```python
from build123d import *

# Parameters (mm, degrees)
SKETCH_1_R                       = 1.85
SKETCH_1_R_2                     = 32.5
SM_BASE_FLANGE_1_DEPTH           = 3
SM_EDGE_FLANGE_1_STRIP_W         = 13.4732
SM_EDGE_FLANGE_1_STRIP_H         = 3
SM_EDGE_FLANGE_1_STRIP_CUT_DEPTH = 100
SM_EDGE_FLANGE_1_DEPTH           = 100
SKETCH_9_R                       = 2.1
CUT_EXTRUDE_1_DEPTH              = 10
FILLET_1_R                       = 5
SKETCH_10_R                      = 2.1
CUT_EXTRUDE_2_DEPTH              = 10


# Sheet-metal steps are written as plain solids
with BuildPart() as part:
    # Sketch 1 → 基体-法兰1 (new body)
    with BuildSketch(Plane(origin=(0, 0, 0), x_dir=(0, 0, -1), z_dir=(1, 0, 0))):
        with BuildLine():
            Line((-50, 0), (-50, -55.5))
            Line((-50, -55.5), (50, -55.5))
            Line((50, -55.5), (50, 0))
            ThreePointArc((50, 0), (0, 50), (-50, 0))
        make_face()
        with Locations((0, 42.5)):
            Circle(SKETCH_1_R, mode=Mode.SUBTRACT)
        with Locations((30.0520382, 30.0520382)):
            Circle(SKETCH_1_R, mode=Mode.SUBTRACT)
        with Locations((42.5, 0)):
            Circle(SKETCH_1_R, mode=Mode.SUBTRACT)
        with Locations((30.0520382, -30.0520382)):
            Circle(SKETCH_1_R, mode=Mode.SUBTRACT)
        with Locations((0, -42.5)):
            Circle(SKETCH_1_R, mode=Mode.SUBTRACT)
        with Locations((-30.0520382, -30.0520382)):
            Circle(SKETCH_1_R, mode=Mode.SUBTRACT)
        with Locations((-42.5, 0)):
            Circle(SKETCH_1_R, mode=Mode.SUBTRACT)
        with Locations((-30.0520382, 30.0520382)):
            Circle(SKETCH_1_R, mode=Mode.SUBTRACT)
        Circle(SKETCH_1_R_2, mode=Mode.SUBTRACT)
    extrude(amount=-SM_BASE_FLANGE_1_DEPTH)

    # 边线-法兰1 strip (across the edge) → 边线-法兰1 strip cut (cut)
    with BuildSketch(Plane(origin=(-3, -55.5, -50), x_dir=(0, 1, 0), z_dir=(0, 0, 1))):
        with Locations((-3, -1.5)):
            Rectangle(SM_EDGE_FLANGE_1_STRIP_W, SM_EDGE_FLANGE_1_STRIP_H)
    extrude(amount=SM_EDGE_FLANGE_1_STRIP_CUT_DEPTH, mode=Mode.SUBTRACT)

    # 边线-法兰1 section (across the edge) → 边线-法兰1 (add)
    with BuildSketch(Plane(origin=(-3, -55.5, -50), x_dir=(0, 1, 0), z_dir=(0, 0, 1))):
        with BuildLine():
            Line((0, 0.7366), (0, 50))
            Line((0, 50), (3, 50))
            Line((3, 50), (3, 0.7366))
            ThreePointArc((3, 0.7366), (3.215745145, 0.215745145), (3.7366, 0))
            Line((3.7366, 0), (3.7366, -3))
            ThreePointArc((3.7366, -3), (1.094424801, -1.905575199), (0, 0.7366))
        make_face()
    extrude(amount=SM_EDGE_FLANGE_1_DEPTH)

    # 草图9 → 切除-拉伸1 (cut)
    with BuildSketch(Plane(origin=(0, -52.5, 0), x_dir=(1, 0, 0), z_dir=(0, 1, 0))):
        with Locations(Location((-45.5, 42.5, 0), (0, 0, 180))):
            Circle(SKETCH_9_R)
        with Locations(Location((-10.5, 42.5, 0), (0, 0, 180))):
            Circle(SKETCH_9_R)
        with Locations(Location((-45.5, -42.5, 0), (0, 0, 180))):
            Circle(SKETCH_9_R)
        with Locations(Location((-10.5, -42.5, 0), (0, 0, 180))):
            Circle(SKETCH_9_R)
    extrude(amount=-CUT_EXTRUDE_1_DEPTH, mode=Mode.SUBTRACT)

    # 圆角1
    fillet_1_edges = [part.edges().sort_by_distance(p)[0] for p in [
        (-53, -54, -50),
        (-53, -54, 50),
    ]]
    fillet(fillet_1_edges, radius=FILLET_1_R)

    # 草图10 → 切除-拉伸2 (cut)
    with BuildSketch(Plane(origin=(0, -52.5, 0), x_dir=(1, 0, 0), z_dir=(0, 1, 0))):
        with Locations(Location((-28, 0, 0), (0, 0, 180))):
            Circle(SKETCH_10_R)
        with BuildLine():
            Line((-43.4, 22.5), (-43.4, -22.5))
            ThreePointArc((-43.4, -22.5), (-45.5, -24.6), (-47.6, -22.5))
            Line((-47.6, -22.5), (-47.6, 22.5))
            ThreePointArc((-47.6, 22.5), (-45.5, 24.6), (-43.4, 22.5))
        make_face()
        with BuildLine():
            Line((-8.4, 22.5), (-8.4, -22.5))
            ThreePointArc((-8.4, -22.5), (-10.5, -24.6), (-12.6, -22.5))
            Line((-12.6, -22.5), (-12.6, 22.5))
            ThreePointArc((-12.6, 22.5), (-10.5, 24.6), (-8.4, 22.5))
        make_face()
    extrude(amount=-CUT_EXTRUDE_2_DEPTH, mode=Mode.SUBTRACT)


solid = part.part
```
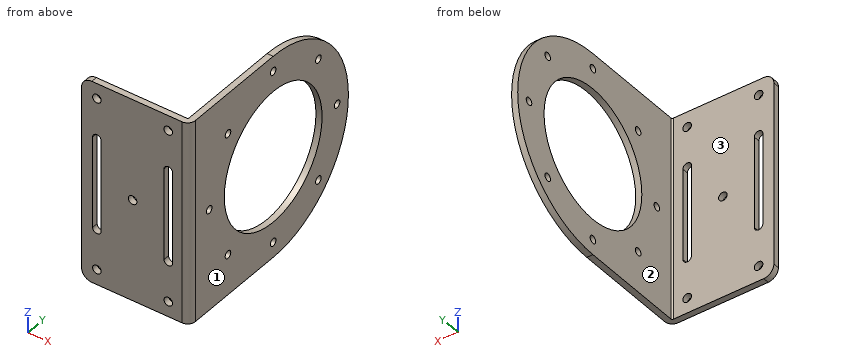
Can you work these out from the model? Positions are in its coordinate system, mm. Face numbers are marked on the shaded views. Round coordinates to 2 decimals unless told otherwise and drop trailing zeros. Order: outer loops, then holes, each group sorted by start corner. A loop starts at its lowest first (then second) coordinate and runs counter-clockwise, first axis right, second up.
(1) If we section it at C-C (z = 0): Count the separate pieces of the cut face and the enclosed holes in it, plus the area to 3 significant figures.
Results are:
separate pieces: 7
enclosed holes: 0
area: 209 mm2
(2) If we section it at D-D (x = -10.5): Please give me the cut outline in (y, z).
Results are:
outline: (-55.5, -50) - (-52.5, -50) - (-52.5, -44.6) - (-55.5, -44.6) - close; (-55.5, -40.4) - (-52.5, -40.4) - (-52.5, -24.6) - (-55.5, -24.6) - close; (-55.5, 24.6) - (-52.5, 24.6) - (-52.5, 40.4) - (-55.5, 40.4) - close; (-55.5, 44.6) - (-52.5, 44.6) - (-52.5, 50) - (-55.5, 50) - close
(3) If we section it at A-A (y = -42.5): Please give me the cut outline in (x, z), plus the area to 3 significant figures.
Results are:
outline: (-3, -50) - (0, -50) - (0, -1.85) - (-3, -1.85) - close; (-3, 1.85) - (0, 1.85) - (0, 50) - (-3, 50) - close
area: 289 mm2
(4) I'm going to push flat-ended pins straight in: pin 1 (5 mm diameter, centred on x = -40, z = -18, fed in from +Y); pin 2 (3.5 mm diameter, centred on y = -54, z = 0.5, fed in from +X); pin 3 (5 mm diameter, centred on y = -30.05, z = -30.05, fed in from -X). Where does each tip first touch, or does it pass through?
Results are:
pin 1: stops at y = -52.5
pin 2: stops at x = -0.03
pin 3: stops at x = -3
(5) If I drill on L1, parallel to X at y = -54, z = 42; L2, parallel to Y at x = -24.5, z = 9; L3, parallel to X at y = -41.5, z = 32.5, over which ranges is the centre line in solid material (lowest first)?
Results are:
L1: x = -53 to -47.54, -43.46 to -12.54, -8.46 to -0.74
L2: y = -55.5 to -52.5
L3: x = -3 to 0
(6) If we section it at B-B (x = -28): Please give me the cut outline in (y, z), plus the area to 3 significant figures.
Results are:
outline: (-55.5, -50) - (-52.5, -50) - (-52.5, -2.1) - (-55.5, -2.1) - close; (-55.5, 2.1) - (-52.5, 2.1) - (-52.5, 50) - (-55.5, 50) - close
area: 287 mm2
(7) We'd pull the mould along X, two halves only. Please class the marked faces 1, 2 and 3: +X half, -X half, draft (parallel to the pull), parting line (faces both ways), or undercut.
Results are:
face 1: +X half
face 2: -X half
face 3: draft
